```python
from build123d import *

# Parameters (mm, degrees)
SKETCH_1_W          = 20
SKETCH_1_H          = 50
SKETCH_1_W_2        = 17
SKETCH_1_H_2        = 47
EXTRUDE_1_DEPTH     = 250
SKETCH_2_R          = 2.5
CUT_EXTRUDE_1_DEPTH = 253.041663223
SKETCH_3_R          = 2.1
CUT_EXTRUDE_2_DEPTH = 256.147016443
SKETCH_4_R          = 1.6
CUT_EXTRUDE_3_DEPTH = 10
SKETCH_5_R          = 4
CUT_EXTRUDE_4_DEPTH = 10
SKETCH_6_R          = 7.5
CUT_EXTRUDE_5_DEPTH = 10
SKETCH_7_R          = 2
CUT_EXTRUDE_6_DEPTH = 253.041663223


with BuildPart() as part:
    # 草图1 → 凸台-拉伸1 (new body)
    with BuildSketch(Plane.XY):
        Rectangle(SKETCH_1_W, SKETCH_1_H)
        Rectangle(SKETCH_1_W_2, SKETCH_1_H_2, mode=Mode.SUBTRACT)
    extrude(amount=-EXTRUDE_1_DEPTH)

    # 草图2 → 切除-拉伸1 (cut, through all)
    with BuildSketch(Plane.ZY.offset(10)):
        with Locations((-56, 12)):
            Circle(SKETCH_2_R)
        with Locations(Location((-97, 12, 0), (0, 0, 180))):
            Circle(SKETCH_2_R)
        with Locations((-97, -18)):
            Circle(SKETCH_2_R)
        with Locations(Location((-56, -18, 0), (0, 0, 180))):
            Circle(SKETCH_2_R)
        with Locations((-194, -18)):
            Circle(SKETCH_2_R)
        with Locations(Location((-153, -18, 0), (0, 0, 180))):
            Circle(SKETCH_2_R)
        with Locations((-153, 12)):
            Circle(SKETCH_2_R)
        with Locations(Location((-194, 12, 0), (0, 0, 180))):
            Circle(SKETCH_2_R)
    extrude(amount=-CUT_EXTRUDE_1_DEPTH, mode=Mode.SUBTRACT)

    # 草图3 → 切除-拉伸2 (cut, through all)
    with BuildSketch(Plane(origin=(0, 25, 0), x_dir=(1, 0, 0), z_dir=(0, 1, 0))):
        with Locations(Location((0, 22.5, 0), (0, 0, 270))):
            Circle(SKETCH_3_R)
        with Locations(Location((0, 7.5, 0), (0, 0, 270))):
            Circle(SKETCH_3_R)
        with Locations(Location((0, 242.5, 0), (0, 0, 90))):
            Circle(SKETCH_3_R)
        with Locations(Location((0, 227.5, 0), (0, 0, 90))):
            Circle(SKETCH_3_R)
    extrude(amount=-CUT_EXTRUDE_2_DEPTH, mode=Mode.SUBTRACT)

    # 草图4 → 切除-拉伸3 (cut)
    with BuildSketch(Plane(origin=(0, 25, 0), x_dir=(1, 0, 0), z_dir=(0, 1, 0))):
        with Locations(Location((0, 130, 0), (0, 0, 270))):
            Circle(SKETCH_4_R)
        with Locations(Location((0, 120, 0), (0, 0, 270))):
            Circle(SKETCH_4_R)
    extrude(amount=-CUT_EXTRUDE_3_DEPTH, mode=Mode.SUBTRACT)

    # 草图5 → 切除-拉伸4 (cut)
    with BuildSketch(Plane(origin=(0, 25, 0), x_dir=(1, 0, 0), z_dir=(0, 1, 0))):
        with Locations(Location((0, 22.5, 0), (0, 0, 270))):
            Circle(SKETCH_5_R)
        with Locations(Location((0, 7.5, 0), (0, 0, 270))):
            Circle(SKETCH_5_R)
        with Locations(Location((0, 242.5, 0), (0, 0, 270))):
            Circle(SKETCH_5_R)
        with Locations(Location((0, 227.5, 0), (0, 0, 270))):
            Circle(SKETCH_5_R)
    extrude(amount=-CUT_EXTRUDE_4_DEPTH, mode=Mode.SUBTRACT)

    # 草图6 → 切除-拉伸5 (cut)
    with BuildSketch(Plane.ZY.offset(10)):
        with Locations((-125, -4)):
            Circle(SKETCH_6_R)
    extrude(amount=-CUT_EXTRUDE_5_DEPTH, mode=Mode.SUBTRACT)

    # 草图7 → 切除-拉伸6 (cut, through all)
    with BuildSketch(Plane.ZY.offset(10)):
        with Locations((-235, 15)):
            Circle(SKETCH_7_R)
        with Locations((-213, 15)):
            Circle(SKETCH_7_R)
        with Locations((-235, -15)):
            Circle(SKETCH_7_R)
        with Locations((-213, -15)):
            Circle(SKETCH_7_R)
        with Locations(Location((-37, -15, 0), (0, 0, 180))):
            Circle(SKETCH_7_R)
        with Locations(Location((-15, -15, 0), (0, 0, 180))):
            Circle(SKETCH_7_R)
        with Locations(Location((-37, 15, 0), (0, 0, 180))):
            Circle(SKETCH_7_R)
        with Locations(Location((-15, 15, 0), (0, 0, 180))):
            Circle(SKETCH_7_R)
    extrude(amount=-CUT_EXTRUDE_6_DEPTH, mode=Mode.SUBTRACT)


solid = part.part
```
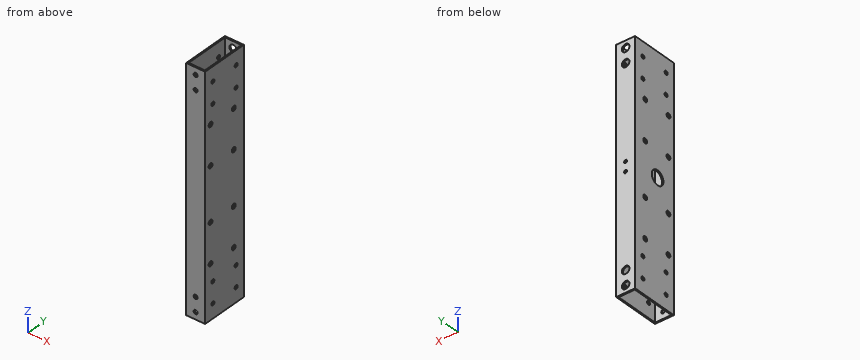
Check sheet for the modelled part. Datum: model origin and axes. Units: mm. Coordinates: 2 decimals unless noted, no trailing zeros. Loops run counter-clockwise (first coordinate to the right, second up) from the corner with the lowest first, then second, coordinate; pieces in that order, holes last. Notation, with made-up numbers: M -27.75,-1 L -11.75,-1 A24 cw -11.75,37 Z; hole C -7.75,84 d2. An arc over 180 degrees is marked long. Answer as a JSON object with one key per item and string values.
1. Sectioned sample at B-B on z = -169. Record the cut outline in (x, y), and give its area (3 significant figures).
Outcome:
{"outline": "M -10,-25 L 10,-25 L 10,25 L -10,25 Z; hole M -8.5,-23.5 L 8.5,-23.5 L 8.5,23.5 L -8.5,23.5 Z", "area": "201 mm²"}
2. Sectioned sample at A-A on z = -227.5. Record the cut outline in (x, y).
Outcome:
{"outline": "M -10,-25 L -2.1,-25 L -2.1,-23.5 L -8.5,-23.5 L -8.5,23.5 L -4,23.5 L -4,25 L -10,25 Z; M 2.1,-25 L 10,-25 L 10,25 L 4,25 L 4,23.5 L 8.5,23.5 L 8.5,-23.5 L 2.1,-23.5 Z"}
3. Scan lines: L1, parallel to X at y = 9, z = -69.5; L2, parallel to Y at x = -5.25, z = -35; L3, parallel to Y at x = -8.9, z = -125. Record each from-to range of solid material in increasing order. Write a range as from..to.
Outcome:
{"L1": "-10..-8.5, 8.5..10", "L2": "-25..-23.5, 23.5..25", "L3": "-25..-11.5, 3.5..25"}
4. Depth check by flat-ended pin: P1, Ø3.5, axis at x = 0, z = -227.5, coming from the +Y side; P2, Ø1.9, axis at x = 0, z = -130, coming from the +Y side. Enter the tip coordinate at first touch or a pass-through.
Outcome:
{"P1": "through", "P2": "y = -23.5"}
